The figure shows three views and two pictorial views of one solid part (mm, origin at its lowest corner). Answer the questions. Give positions to 0.01 mm unless a question says otherwise; leave off trailing zeros. Order: outer loops, then holes, each group sorted by start corner. A loop starts at its lowest first (then second) coordinate and runs counter-clockwise, first axis right, second up. Notation, with made-up numbers: (58.25, -25) - (103.25, -25) arc R31 cw to (103.25, 1) - close; hole circle Ø9 at (77.5, -22.75). An arc over 180 degrees is marked (long way). Use a Markdown table: item, result. Add a question column.
1. A cutting plane is placed at B-B on x = 56. Determine the outline of the cut face in (y, z).
2. Flat-ended cylindrical pins translate along their axes: P1, Ø0.9, axis at x = 2, z = 1.5, coming from the -Y side; P2, Ø1, axis at x = 62, z = 1.5, coming from the -Y side; P3, Ø1.5, axis at y = 4.5, z = 1, coming from the +X side. Find the tip coordinate at first contact, or state that the pin passes through.
3. A cutting plane is placed at A-A on z = 2.15. Determine the outline of the cut face in (x, y), and give its area (3 significant figures).
4. Consider L1, parallel to X at y = 9, z = 2.15; L2, parallel to Y at x = 44, z = 2.95. Determine where each line is inside the solid, lowest interval first.
5. A cutting plane is placed at C-C on y = 14. Determine the outline of the cut face in (x, z), and give its area (3 significant figures).
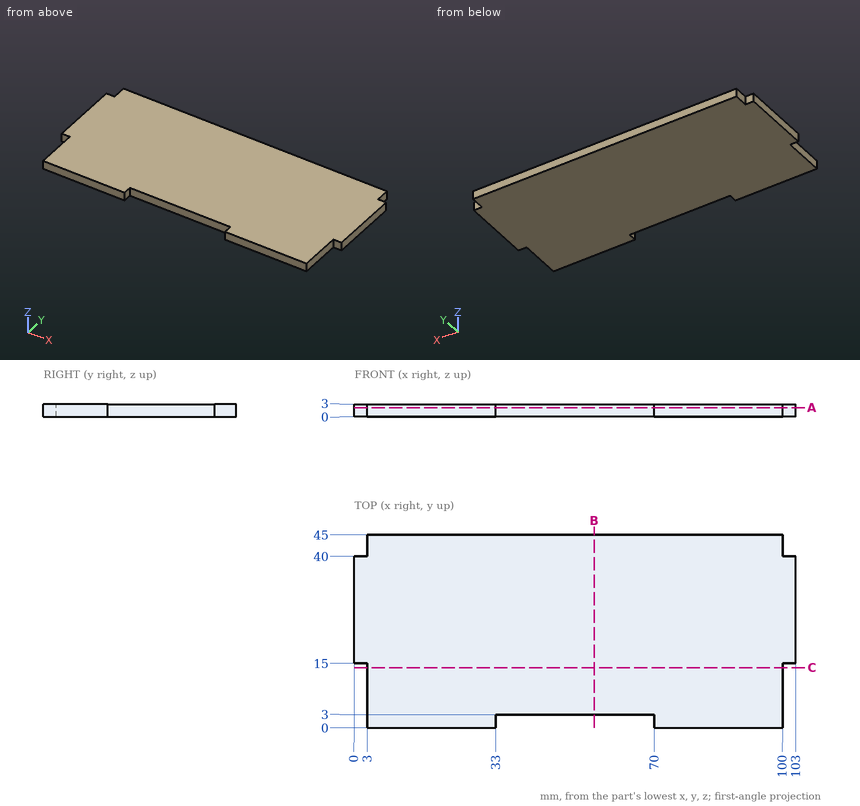
Output values:
| question | item | result |
|---|---|---|
| 1 | outline | (3, 0) - (45, 0) - (45, 3) - (3, 3) - close |
| 2 | P1 | y = 15 |
| 2 | P2 | y = 3 |
| 2 | P3 | x = 100 |
| 3 | outline | (0, 15) - (3, 15) - (3, 0) - (33, 0) - (33, 3) - (70, 3) - (70, 0) - (100, 0) - (100, 15) - (103, 15) - (103, 40) - (100, 40) - (100, 45) - (3, 45) - (3, 40) - (0, 40) - close |
| 3 | area | 4,400 mm² |
| 4 | L1 | 3 to 100 |
| 4 | L2 | 3 to 45 |
| 5 | outline | (3, 0) - (100, 0) - (100, 3) - (3, 3) - close |
| 5 | area | 291 mm² |
